Autodesk Inventor part; units mm, degrees
ref_plane "YZ Plane" through (0, 0, 0) normal (1, 0, 0) x (0, 1, 0)
ref_plane "XZ Plane" through (0, 0, 0) normal (0, 1, 0) x (-1, 0, 0)
ref_plane "XY Plane" through (0, 0, 0) normal (0, 0, 1) x (1, 0, 0)
sketch "Sketch1" plane through (0, 0, 0) normal (0, 0, 1) x (1, 0, 0)
  line L0 (20, -22) -> (4.1, -22) construction
  line L1 (4.1, -22) -> (4.1, -25) construction
  line L2 (4.1, -25) -> (0, -25) construction
  line L3 (30, -47) -> (20, -47) construction
  circle A0 centre (17, -17) radius 3 construction
  line L4 (14, -17) -> (14, 0) construction
  line L5 (14, 0) -> (30, 0) construction
  line L6 (20, -47) -> (20, -17) construction
  line L7 (20, -47) -> (30, -47) construction
  line L8 (30, -47) -> (30, 0) construction
  line L9 (0, -25) -> (0, 0) construction
  line L10 (30, 0) -> (30, -47) construction
  line L11 (-7.0263, 0) -> (42.1581, 0) construction
  line L12 (0, -63.6142) -> (0, 17.6853) construction
  line L13 (17, -17) -> (17, -8) construction
  circle A1 centre (17, -8) radius 3 construction
  line L14 (16.5, -38) -> (20, -38)
  line L15 (16.5, -45) -> (25, -45)
  line L16 (25, -45) -> (29.0415, -52)
  line L17 (29.0415, -52) -> (31, -52)
  line L18 (31, -52) -> (30, -44.4042)
  line L19 (30, -44.4042) -> (30, -1)
  line L20 (15, -1) -> (30, -1)
  line L21 (15, -1) -> (15, -5.7639)
  line L22 (16.5, -45) -> (16.5, -38)
  arc A2 (20, -8) -> (15, -5.7639) centre (17, -8) ccw
  line L23 (20, -8) -> (20, -38)
  line L24 (27, -1) -> (34.0711, 6.0711)
  line L25 (34.0711, 6.0711) -> (35.1317, 5.0104)
  line L26 (30, -6) -> (35.1317, 5.0104)
  point P0 (0, 0)
  point P1 (0, 0)
  dimension "d10" = 6
  dimension "d1" = 3
  dimension "d2" = 5
  dimension "d3" = 14
  dimension "d4" = 20
  dimension "d5" = 22
  dimension "d6" = 30
  dimension "d7" = 4.1
  dimension "d8" = 3
  dimension "d9" = 25
  dimension "d11" = 9
  dimension "d12" = 0
  dimension "d13" = 16
  dimension "d14" = 7
  dimension "d15" = 3.5
  dimension "d16" = 120
  dimension "d17" = 7.5
  dimension "d19" = 5
  dimension "d20" = 5
  dimension "d21" = 1
  dimension "d22" = 1
  dimension "d23" = 1
  dimension "d40" = 45
  dimension "d41" = 3
  dimension "d42" = 10
  dimension "d43" = 5
  dimension "d46" = 1.5
extrude "Extrusion1" add sketch "Sketch1" along normal mid plane 9.8
fillet "Fillet1" radius 0.5 1 edges at (15, -5.7639, 0)
fillet "Fillet2" radius 1 2 edges at (29.0415, -52, 0) (31, -52, 0)
fillet "Fillet3" radius 3 3 edges at (16.5, -45, 0) (25, -45, 0) (30, -44.4042, 0)
fillet "Fillet4" radius 2 1 edges at (15, -1, 0)
fillet "Fillet5" radius 1 1 edges at (20, -38, 0)
sketch "Sketch2" plane through (30, -44.2076, 4.9) normal (1, 0, 0) x (0, 0, -1)
  line L0 (-1.96, 44.2076) -> (11.76, 44.2076) construction
  line L1 (4.9, -19.4066) -> (4.9, 61.8929) construction
  point P0 (4.9, 44.2076)
  point P1 (4.9, 32.2076)
  dimension "d44" = 12
hole "Hole1" at (30, -12, 0) direction (-1, 0, 0) diameter 5 end through all
fillet "Fillet6" radius 2 2 edges at (30, -12, 2.5) (20, -12, 2.5)
fillet "Fillet8" radius 1 2 edges at (34.0711, 6.0711, 0) (35.1317, 5.0104, 0)
fillet "Fillet9" radius 2 1 edges at (27, -1, 0)
fillet "Fillet10" radius 1 1 edges at (16.5, -38, 0)
fillet "Fillet11" radius 2 1 edges at (30, -6, 0)
sketch "Sketch3" plane through (0, 0, 4.9) normal (0, 0, 1) x (1, 0, 0)
  line L0 (-6.9365, 0) -> (41.6191, 0)
  line L1 (20, -8) -> (20, -37)
  point P0 (0, 0)
  point P1 (20, -12.995)
  point P2 (25, -12)
  dimension "d51" = 12
  dimension "d52" = 5
hole "Hole2" at (25, -12, 4.9) direction (0, 0, -1) diameter 5 end through all
properties part number "P104Levier" material "ABS Plastic"
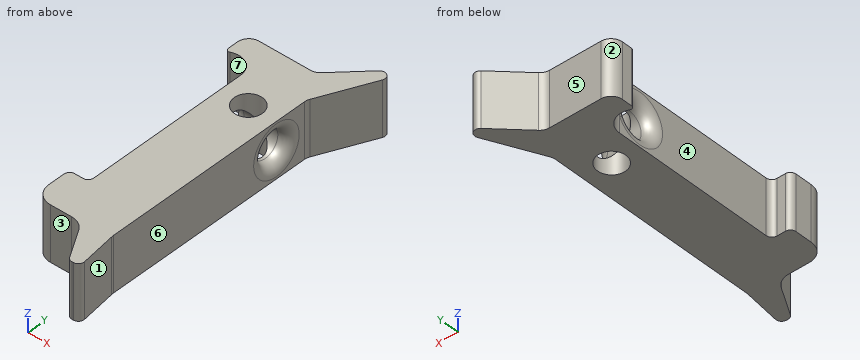
For this review, take the finished solid that the model builds, in its own axes (mm). Face numbers are marked on the shaded views. A direction names the side the tool comes from. Round coordinates to 2 decimals unless told otherwise and drop trailing zeros. Loops run counter-clockwise (first coordinate to the right, second up) from the corner with the lowest first, then second, coordinate; pieces in that order, holes last.
(1) We need section A-A (y = -12). Give the boundary of the cut face in (x, z), plus the area to 3 significant figures.
Returned:
outline: (20, -4.9) - (22.5, -4.9) - (22.5, -2.5) - (22, -2.5) arc R2 ccw to (20, -4.5) - close; (20, 4.5) arc R2 ccw to (22, 2.5) - (22.5, 2.5) - (22.5, 4.9) - (20, 4.9) - close; (27.5, -4.9) - (30, -4.9) - (30, -4.5) arc R2 ccw to (28, -2.5) - (27.5, -2.5) - close; (27.5, 2.5) - (28, 2.5) arc R2 ccw to (30, 4.5) - (30, 4.9) - (27.5, 4.9) - close
area: 20.6 mm2
(2) We need section C-C (x = 31.5). Give the boundary of the cut face in (y, z).
Returned:
outline: (-2.78, -4.9) - (3.5, -4.9) - (3.5, 4.9) - (-2.78, 4.9) - close
(3) Wall thickness on line 1 along Y through (x, z) = (23.5, 0); line 2 along Y through (x, z) = (25.5, 4); line 3 along X through (y, z) = (-8.5, 4): over which ranges is each line inside the solid? List them lowest first.
Returned:
line 1: y = -45.01 to -14.5, -9.5 to -1
line 2: y = -46 to -14.45, -9.55 to -1
line 3: x = 20 to 30
(4) Mouldability with a two-part tool opening along Y and no side actions: class the marked faces 1, 2 and 3 as released by +Y, released by -Y, zero draft, split by the parting line, or undercut.
Returned:
face 1: undercut
face 2: released by +Y
face 3: released by -Y
(5) Clearance check with flat-ended pins moving along their axes: P1, Ø1.6, axis at x = 18.5, z = -2, coming from the +Y side; P2, Ø0.9, axis at y = -41, z = 0, coming from the -X side; P3, Ø3, axis at y = -28.5, z = -2.5, coming from the -X side. State where each tip first meets the part, or that it passes through.
Returned:
P1: stops at y = -1
P2: stops at x = 16.5
P3: stops at x = 20
(6) Tool access review of the marked faces 4, 5, 6 and 7: name each direction out of +Z, -Z, +X, -X, +Y, -Y from which nothing blocks a thin tool from reaching the whole face with its end or side.
Returned:
face 4: +Z, -Z, -X
face 5: +Z, -Z, -X, +Y
face 6: +Z, -Z, +X
face 7: +Z, -Z
(7) We need section B-B (y = -23). Give the boundary of the cut face in (x, z).
Returned:
outline: (20, -4.9) - (30, -4.9) - (30, 4.9) - (20, 4.9) - close
